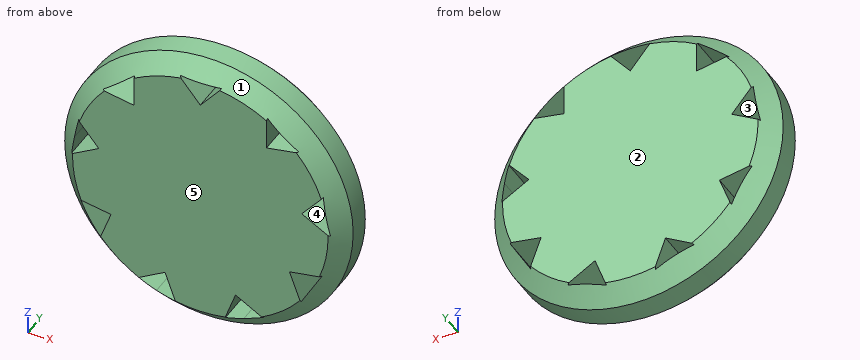
from build123d import *

# Parameters (mm, degrees)
F0_R     = 44.45
F1_DEPTH = 17.272
F3_DEPTH = 17.273


# Not quite as in the source:
# - a fillet or chamfer that OpenCascade refuses, or shapes differently, is made with other operations: its cross-section is extruded or revolved along the edge and cut away or added


with BuildPart() as f1:
    # F0 (on Front) → F1 (new body)
    with BuildSketch(Plane.XZ):
        Circle(F0_R)
    extrude(amount=F1_DEPTH)

    # F2 (on face) → F3 (cut, through all)
    with BuildSketch(Plane.XZ.offset(17.272)):
        Polygon((6.35, 39.37), (0, 39.37), (-6.35, 39.37), (0, 31.75), align=None)
        Polygon((-20.4085066075, 24.321911069), (-20.4421659796, 34.2408710471), (-25.3065481934, 30.1591697256), (-30.1709304072, 26.0774684041), align=None)
        Polygon((-31.2676461581, 5.5133296409), (-37.6692153079, 13.0900579864), (-38.7718812361, 6.8365287547), (-39.8745471643, 0.5829995231), align=None)
        Polygon((-27.4963065702, -15.875), (-37.270420147, -14.185738686), (-34.095420147, -19.685), (-30.920420147, -25.184261314), align=None)
        Polygon((-10.8591395506, -29.83524071), (-19.4323811847, -34.8238705702), (-13.4653330427, -36.9956984803), (-7.4982849007, -39.1675263905), align=None)
        Polygon((10.8591395506, -29.83524071), (7.4982849007, -39.1675263905), (13.4653330427, -36.9956984803), (19.4323811847, -34.8238705702), align=None)
        Polygon((27.4963065702, -15.875), (30.920420147, -25.184261314), (34.095420147, -19.685), (37.270420147, -14.185738686), align=None)
        Polygon((31.2676461581, 5.5133296409), (39.8745471643, 0.5829995231), (38.7718812361, 6.8365287547), (37.6692153079, 13.0900579864), align=None)
        Polygon((20.4085066075, 24.321911069), (30.1709304072, 26.0774684041), (25.3065481934, 30.1591697256), (20.4421659796, 34.2408710471), align=None)
    extrude(amount=-F3_DEPTH, mode=Mode.SUBTRACT)

    # F4: chamfer of 5.08 on 2 edges, made by hand

    # F4_s1 → F4_t2 (revolve, cut)
    with BuildSketch(Plane.XY):
        Polygon((44.45, -12.192), (39.37, -17.272), (44.45, -17.272), align=None)
    revolve(axis=Axis((0, -17.272, 0), (0, -1, 0)), mode=Mode.SUBTRACT)

    # F4_s3 → F4_t4 (revolve, cut)
    with BuildSketch(Plane.XY):
        Polygon((44.45, -5.08), (39.37, 0), (44.45, 0), align=None)
    revolve(axis=Axis((0, 0, 0), (0, -1, 0)), mode=Mode.SUBTRACT)


solid = f1.part
The listing builds one solid part. Answer for the finished solid, in the listing's coordinates (mm). Face numbers are marked on the shaded views. A direction names the side the tool comes from. Coordinates: 2 decimals unless noted, no trailing zeros. Put each result on its own line as item: value.
1. Flat-ended cylindrical pins translate along their axes: pin 1 Ø10 at (x, y) = (-1, -7) entering from -Z; pin 2 Ø4 at (y, z) = (-4, -28.5) entering from -X; pin 3 Ø6 at (x, y) = (7.5, -9.5) entering from +Z. Find the tip coordinate at first contact, or state that the pin passes through.
Answer sheet:
pin 1: stops at z = -44.45
pin 2: stops at x = -35.45
pin 3: stops at z = 44.22
2. A tool of negligible diameter and unlimited length cuts with its end or side. For the marked faces 4 and 5, from which of +Z, -Z, +X, -X, +Y, -Y can it reach the whole face along a straight path? Write none if from no direction.
Answer sheet:
face 4: +Y, -Y
face 5: +Z, -Z, +X, -X, -Y
3. Find the intervals of material crossed by line 1 along X through (y, z) = (-11.5, -34); line 2 along Z through (x, y) = (35.5, -15.5); line 3 along Z through (x, y) = (32, -7.25), in increasing order. Write a range as from..to.
Answer sheet:
line 1: x = -28.63..-18.02, -9.36..9.36, 18.02..28.63
line 2: z = -20.79..-17.25, -14.49..3.09, 10.52..20.79
line 3: z = -30.85..-23.31, -15.1..5.09, 6.38..30.85
4. The part is cut by section A-A on y = -7.75. State how many separate pieces and enclosed holes the cut face has, plus the area to 3 significant figures.
Answer sheet:
separate pieces: 1
enclosed holes: 9
area: 5,770 mm^2
5. Determine the mould class of the marked faces 1, 2 and 3 for opening direction Z: pulls with the +Z half, pulls with the -Z half, needs draft (parallel to the pull), parting line crosses it, or undercut.
Answer sheet:
face 1: parting line crosses it
face 2: needs draft
face 3: undercut
